from build123d import *

# Parameters (mm, degrees)
ESQUISSE1_R             = 2
BOSS_EXTRU_1_DEPTH      = 2
BOSS_EXTRU_2_DEPTH      = 2
BOSS_EXTRU_3_REACH      = 67.218
ENL_V_MAT_EXTRU_5_DEPTH = 66.43216575
CONG_1_R                = 1
CONG_2_R                = 1


with BuildPart() as part:
    # Esquisse1 → Boss.-Extru.1 (new body)
    with BuildSketch(Plane.XY):
        with BuildLine():
            Line((0, -6), (16, -6))
            ThreePointArc((16, -6), (19.434160723, -4.920014241), (21.632039887, -2.06884671))
            Line((21.632039887, -2.06884671), (22.429477002, 0.102023476))
            ThreePointArc((22.429477002, 0.102023476), (23.818382286, 2.656840718), (25.883595813, 4.704044206))
            Line((25.883595813, 4.704044206), (43.907312567, 17.986833146))
            Line((43.907312567, 17.986833146), (60.52335338, 21.579490619))
            Line((60.52335338, 21.579490619), (60, 24))
            Line((60, 24), (23, 16))
            Line((23, 16), (23, 14))
            Line((23, 14), (-1.899172411, 5.691497532))
            ThreePointArc((-1.899172411, 5.691497532), (-5.92237221, -0.962032954), (0, -6))
        make_face()
        Circle(ESQUISSE1_R, mode=Mode.SUBTRACT)
        with Locations((16, 0)):
            Circle(ESQUISSE1_R, mode=Mode.SUBTRACT)
    boss_extru_1 = extrude(amount=BOSS_EXTRU_1_DEPTH)

    # Esquisse2 → Boss.-Extru.2 (add)
    with BuildSketch(Plane(origin=(0, 0, 0), x_dir=(-1, 0, 0), z_dir=(0, 0, -1))):
        Polygon((-60.52335338, 21.579490619), (-60, 24), (-23, 16), (-23, 14), align=None)
    boss_extru_2 = extrude(amount=BOSS_EXTRU_2_DEPTH)

    # Symétrie1: Boss.-Extru.1, Boss.-Extru.2 across plane
    add(boss_extru_1.mirror(Plane.XY.offset(-2)))
    add(boss_extru_2.mirror(Plane.XY.offset(-2)))

    # Boss.-Extru.3: up to this plane
    boss_extru_3_end = Plane(origin=(23, 14, -2), z_dir=(-0.19799508496371696, 0.9802030128142897, 0))
    # Esquisse7 → Boss.-Extru.3 (add, up to the surface)
    with BuildSketch(Plane(origin=(-2.277739009, 10.534542917, 0), x_dir=(0.9774141654398673, 0.21133279252753906, 0), z_dir=(-0.21133279252753906, 0.9774141654398673, 0)), mode=Mode.PRIVATE) as boss_extru_3_sk1:
        Polygon((25.861850486, -2), (63.667267202, -3.999795233), (63.716836947, 2), (63.716836947, 8), (25.861850486, 6), align=None)
    boss_extru_3_tool1 = split(extrude(boss_extru_3_sk1.sketch, amount=-BOSS_EXTRU_3_REACH, mode=Mode.PRIVATE), bisect_by=boss_extru_3_end, keep=Keep.BOTH, mode=Mode.PRIVATE)
    add(boss_extru_3_tool1.solids().sort_by_distance((42.727149, 20.265329, -2.000928))[0])

    # Esquisse8 → Enlèv. mat.-Extru.5 (cut, through all)
    with BuildSketch(Plane(origin=(-2.277739009, 10.534542917, 0), x_dir=(0.9774141654398673, 0.21133279252753906, 0), z_dir=(-0.21133279252753906, 0.9774141654398673, 0))):
        with BuildLine():
            Line((57.893179092, 7.823657855), (58.153804594, 10.152084359))
            Line((58.153804594, 10.152084359), (67.029835538, 10.152084359))
            Line((67.029835538, 10.152084359), (67.337455885, -6.822766653))
            Line((67.337455885, -6.822766653), (57.261437216, -6.223219))
            Line((57.261437216, -6.223219), (57.893179092, -3.823657855))
            ThreePointArc((57.893179092, -3.823657855), (63.716836947, 2), (57.893179092, 7.823657855))
        make_face()
    extrude(amount=-ENL_V_MAT_EXTRU_5_DEPTH, mode=Mode.SUBTRACT)

    # Congé1
    cong_1_edges = [part.edges().sort_by_distance(p)[0] for p in [
        (41.588067586, 17.75467732, -4),
        (41.588067586, 17.75467732, 0),
    ]]
    fillet(cong_1_edges, radius=CONG_1_R)

    # Congé2
    # the kernel refuses this fillet: 1 mm, written as the material it takes off along each edge
    with BuildSketch(Plane(origin=(57.690537844, 23.500656831, -7.875164208), x_dir=(0.21133279252753906, -0.9774141654398673, 0), z_dir=(-0.9760528637131802, -0.21103845701906618, 0.05275961425476653))) as cong_2_piece_1_section:
        with BuildLine():
            CenterArc((CONG_2_R, CONG_2_R), CONG_2_R, 180, 90)
            Line((0, CONG_2_R), (0, 0))
            Line((0, 0), (CONG_2_R, 0))
        make_face()
    cong_2_piece_1 = extrude(amount=38.041658791, mode=Mode.PRIVATE)
    cong_2_piece_1 = split(cong_2_piece_1, bisect_by=Plane(origin=(54.069822656, 22.51805355, -6), z_dir=(0, 0, -1)), keep=Keep.TOP, mode=Mode.PRIVATE)
    add(cong_2_piece_1, mode=Mode.SUBTRACT)
    with BuildSketch(Plane(origin=(20.559876055, 15.472405634, 1.867941987), x_dir=(0.2113327925275391, -0.9774141654398673, 0), z_dir=(0.9760495779057013, 0.2110377465742059, 0.05282320504270329))) as cong_2_piece_2_section:
        with BuildLine():
            CenterArc((CONG_2_R, CONG_2_R), CONG_2_R, 180, 90)
            Line((0, CONG_2_R), (0, 0))
            Line((0, 0), (CONG_2_R, 0))
        make_face()
    cong_2_piece_2 = extrude(amount=38.032176769, mode=Mode.PRIVATE)
    cong_2_piece_2 = split(cong_2_piece_2, bisect_by=Plane(origin=(39.441724265, 19.308611578, 2), z_dir=(0, 0, 1)), keep=Keep.TOP, mode=Mode.PRIVATE)
    add(cong_2_piece_2, mode=Mode.SUBTRACT)


solid = part.part
Work out the finished part from the listing and answer in its coordinate system (mm). A direction names the side the tool comes from. Round coordinates to 2 decimals unless told otherwise and drop trailing zeros. Order: outer loops, then holes, each group sorted by start corner. A loop starts at its lowest first (then second) coordinate and runs counter-clockwise, first axis right, second up. Notation, with made-up numbers: M 42.25,21.5 L 53.25,21.5 A21 ccw 53.25,59.5 Z; hole C 74,69.5 d2. An arc over 180 degrees is marked long. Put each result on its own line as item: value. Start each with the question number.
Q1. A tool of negligible diameter and unlimited length cuts with its end or side. For faces 1 (the cylindrical face through (33.078, 15.745, -3.699)), 2 (the flat face through (44.89, 18.42, -6.69)), 3 (the cylindrical face through (14.4, -1.2, 1)), from which of +Z, -Z, +X, -X, +Y, -Y can it reach the whole face along a straight path? Write none if from no direction.
Q2. For a pull along Z with two mould halves and no side action, classify faces 4 (the cylindrical face through (60.257, 22.806, -1.881)), 5 (the flat face through (8, -6, -5)), 6 (the flat face through (41.499, 17.737, -2.014)), 7 (the flat face through (12, 3, -4)) as pulls with the +Z half, pulls with the -Z half, needs draft (parallel to the pull), parting line crosses it, or undercut.
Q3. Flat-ended cylindrical pins translate along their axes: pin 1 (12 mm diameter, centred on x = 20.5, y = 17, fed in from -Z); pin 2 (3 mm diameter, centred on x = 16, y = 0, fed in from +Z); pin 3 (4.5 mm diameter, centred on x = 0, y = 0, fed in from +Z); pin 4 (7 mm diameter, centred on x = 26, y = 8.5, fed in from -Z). Find the tip coordinate at first contact, or state that the pin passes through.
Q4. Straight lines are drawn through the part: L1, parallel to Z at x = 23, y = 3; L2, parallel to X at y = 1, z = 0.5; L3, parallel to Y at x = 16, z = 1.1. For each, find the intervals that lie inside material, in ascending order. Write a range as [from, to].
Q5. Section A-A, the plane y = 3 is taken. Write down the section's boundary in (x, z).
Q6. Section B-B, the plane y = 10 is taken. Write down the section's boundary in (x, z), and give its area (3 significant figures).
Findings below:
1. face 1: +X, -Y
1. face 2: -Z, +X, -Y
1. face 3: +Z, -Z
2. face 4: parting line crosses it
2. face 5: needs draft
2. face 6: undercut
2. face 7: undercut
3. pin 1: stops at z = -6.17
3. pin 2: passes through
3. pin 3: stops at z = 2
3. pin 4: stops at z = -6
4. L1: z = [-6, -4], [0, 2]
4. L2: x = [-5.92, -1.73], [1.73, 14.27], [17.73, 22.81]
4. L3: y = [-6, -2], [2, 11.66]
5. outline: M -5.2,-6 L 24.09,-6 L 24.09,-4 L -5.2,-4 Z; M -5.2,0 L 24.09,0 L 24.09,2 L -5.2,2 Z
6. outline: M 11.01,-6 L 33.07,-6 L 33.07,-4 L 11.01,-4 Z; M 11.01,0 L 33.07,0 L 33.07,2 L 11.01,2 Z
6. area: 88.2 mm^2
